Read the model definition and answer for the solid it produces. Units are mm, in the model's axes. Face numbers are marked on the shaded views. A direction names the side the tool comes from. Round coordinates to 2 decimals unless told otherwise and drop trailing zeros. Loops run counter-clockwise (first coordinate to the right, second up) from the corner with the lowest first, then second, coordinate; pieces in that order, holes last. Notation, with made-up numbers: M 58.5,32.25 L 115.5,32.25 A18 cw 115.5,36.25 Z; hole C 6.5,83 d4. An arc over 180 degrees is marked long. Write each question's results on one line, items separated by ' | '.
```python
from build123d import *

# Parameters (mm, degrees)
SKETCH1_R           = 205
SKETCH1_R_2         = 195
BOSS_EXTRUDE1_DEPTH = 110
CUT_EXTRUDE1_START  = 41.95
CUT_EXTRUDE1_DEPTH  = 26.1
BOSS_EXTRUDE3_DEPTH = 110
SKETCH5_R           = 10
CUT_EXTRUDE2_DEPTH  = 140
FILLET1_R           = 12.5
CUT_EXTRUDE4_START  = -7.5
CUT_EXTRUDE4_DEPTH  = 7.5
CUT_EXTRUDE5_DEPTH  = 7.5
FILLET2_R           = 12.5


with BuildPart() as part:
    # Sketch1 → Boss-Extrude1 (new body)
    with BuildSketch(Plane(origin=(0, 0, 0), x_dir=(0, 0, -1), z_dir=(1, 0, 0))):
        Circle(SKETCH1_R)
        Circle(SKETCH1_R_2, mode=Mode.SUBTRACT)
    extrude(amount=BOSS_EXTRUDE1_DEPTH)

    # Sketch3 → Cut-Extrude1 (cut)
    with BuildSketch(Plane(origin=(0, 0, 0), x_dir=(0, 0, -1), z_dir=(1, 0, 0)).offset(CUT_EXTRUDE1_START)):
        with BuildLine():
            Line((160.8479694, 127.09418059), (137.885822331, 137.885822331))
            ThreePointArc((137.885822331, 137.885822331), (143.004745144, 132.569388874), (147.918824855, 127.063060145))
            Line((147.918824855, 127.063060145), (167.43543162, 118.280920855))
            ThreePointArc((167.43543162, 118.280920855), (164.200841146, 122.731755332), (160.8479694, 127.09418059))
        make_face()
    extrude(amount=CUT_EXTRUDE1_DEPTH, mode=Mode.SUBTRACT)

    # Sketch4 → Boss-Extrude3 (add)
    with BuildSketch(Plane.ZY):
        with BuildLine():
            Line((-339.535373084, 38.097443801), (-170.172659449, 114.307768661))
            ThreePointArc((-170.172659449, 114.307768661), (-156.650879802, -132.232756371), (84.122100255, -186.945104907))
            Line((84.122100255, -186.945104907), (-183.982931916, -307.587784512))
            Line((-183.982931916, -307.587784512), (-339.535373084, 38.097443801))
        make_face()
    extrude(amount=-BOSS_EXTRUDE3_DEPTH)

    # Sketch5 → Cut-Extrude2 (cut)
    with BuildSketch(Plane(origin=(0, -120.642679605, -268.105032171), x_dir=(-1, 0, 0), z_dir=(0, -0.41035170855993064, -0.9119273410102067))):
        with Locations(Location((-90, -185, 0), (0, 0, 90))):
            Circle(SKETCH5_R)
        with Locations(Location((-20, -185, 0), (0, 0, 90))):
            Circle(SKETCH5_R)
        with Locations(Location((-20, 154.071021086, 0), (0, 0, 90))):
            Circle(SKETCH5_R)
        with Locations(Location((-90, 154.071021086, 0), (0, 0, 90))):
            Circle(SKETCH5_R)
    extrude(amount=-CUT_EXTRUDE2_DEPTH, mode=Mode.SUBTRACT)

    # Fillet1
    fillet1_edges = [part.edges().sort_by_distance(p)[0] for p in [
        (55, 114.307768661, -170.172659449),
    ]]
    fillet(fillet1_edges, radius=FILLET1_R)

    # Sketch6 → Cut-Extrude4 (cut)
    with BuildSketch(Plane(origin=(110, 0, 0), x_dir=(0, 0, -1), z_dir=(1, 0, 0)).offset(CUT_EXTRUDE4_START)):
        with BuildLine():
            Line((326.312582588, 33.081687477), (179.407480032, 99.186471399))
            ThreePointArc((179.407480032, 99.186471399), (170.629059775, -113.625366712), (-22.343234006, -203.778752313))
            Line((-22.343234006, -203.778752313), (178.967175591, -294.364994017))
            Line((178.967175591, -294.364994017), (326.312582588, 33.081687477))
        make_face()
    extrude(amount=CUT_EXTRUDE4_DEPTH, mode=Mode.SUBTRACT)

    # Sketch7 → Cut-Extrude5 (cut)
    with BuildSketch(Plane.ZY):
        with BuildLine():
            Line((-179.407480032, 99.186471399), (-326.312582588, 33.081687477))
            Line((-326.312582588, 33.081687477), (-178.967175591, -294.364994017))
            Line((-178.967175591, -294.364994017), (22.343234006, -203.778752313))
            ThreePointArc((22.343234006, -203.778752313), (-170.629059775, -113.625366712), (-179.407480032, 99.186471399))
        make_face()
    extrude(amount=-CUT_EXTRUDE5_DEPTH, mode=Mode.SUBTRACT)

    # Fillet2
    # the kernel refuses this fillet: 12.5 mm, written as the material it adds along each edge
    with BuildSketch(Plane(origin=(102.5, -192.025828775, 48.461834434), x_dir=(1, 0, 0), z_dir=(0, -0.4103517085599303, -0.9119273410102069))) as fillet2_piece_1_section:
        with BuildLine():
            CenterArc((12.5, -11.456439237), FILLET2_R, 113.578178478, 66.421821522)
            Line((0, -11.456439237), (0, 0))
            Line((0, 0), (7.5, 0))
        make_face()
    fillet2_piece_1 = extrude(amount=249.39378369, mode=Mode.PRIVATE)
    fillet2_piece_1 = fillet2_piece_1 - Plane(origin=(104.520833168, 0, 0), x_dir=(0, 0.4838364458471492, -0.8751584391811569), z_dir=(-1, 0, 0)) * Cylinder(205, 545, mode=Mode.PRIVATE)
    add(fillet2_piece_1)
    with BuildSketch(Plane(origin=(102.5, 0, 0), x_dir=(0, 0.6010821181754732, -0.7991872666713895), z_dir=(0, 0.7991872666713895, 0.6010821181754732))) as fillet2_piece_2_section:
        with BuildLine():
            CenterArc((216.456439237, -12.5), FILLET2_R, 90, 66.421821522)
            Line((216.456439237, 0), (205, 0))
            Line((205, 0), (205, -7.5))
        make_face()
    fillet2_piece_2 = revolve(axis=Axis((102.5, 0, 0), (-1, 0, 0)), revolution_arc=141.215785086, mode=Mode.PRIVATE)
    fillet2_piece_2 = split(fillet2_piece_2, bisect_by=Plane(origin=(104.520833168, -262.670858667, -108.533087047), z_dir=(0, 0.9119273410102068, -0.41035170855993025)), keep=Keep.TOP, mode=Mode.PRIVATE)
    fillet2_piece_2 = split(fillet2_piece_2, bisect_by=Plane(origin=(104.520833168, 64.775822826, -255.878494044), z_dir=(0, -0.9119273410102069, 0.41035170855993014)), keep=Keep.TOP, mode=Mode.PRIVATE)
    add(fillet2_piece_2)
    with BuildSketch(Plane(origin=(102.5, 33.081687477, -326.312582588), x_dir=(1, 0, 0), z_dir=(0, 0.41035170855993014, 0.9119273410102069))) as fillet2_piece_3_section:
        with BuildLine():
            CenterArc((12.5, -11.456439237), FILLET2_R, 113.578178478, 66.421821522)
            Line((0, -11.456439237), (0, 0))
            Line((0, 0), (7.5, 0))
        make_face()
    fillet2_piece_3 = extrude(amount=189.734088675, mode=Mode.PRIVATE)
    fillet2_piece_3 = fillet2_piece_3 - Plane(origin=(104.520833168, 0, 0), x_dir=(0, 0.4838364458471492, -0.8751584391811569), z_dir=(-1, 0, 0)) * Cylinder(205, 426, mode=Mode.PRIVATE)
    add(fillet2_piece_3)
    with BuildSketch(Plane(origin=(102.5, -294.364994017, -178.967175591), x_dir=(1, 0, 0), z_dir=(0, 0.9119273410102068, -0.4103517085599305)), Plane(origin=(7.5, 33.081687477, -326.312582588), x_dir=(-1, 0, 0), z_dir=(0, -0.9119273410102068, 0.41035170855993064))) as fillet2_piece_4:
        with BuildLine():
            CenterArc((12.5, -11.456439237), FILLET2_R, 113.578178478, 66.421821522)
            Line((0, -11.456439237), (0, 0))
            Line((0, 0), (7.5, 0))
        make_face()
    extrude(amount=359.071021086)
    with BuildSketch(Plane(origin=(7.5, -294.364994017, -178.967175591), x_dir=(-1, 0, 0), z_dir=(0, 0.41035170855993075, 0.9119273410102067))) as fillet2_piece_5_section:
        with BuildLine():
            CenterArc((12.5, -11.456439237), FILLET2_R, 113.578178478, 66.421821522)
            Line((0, -11.456439237), (0, 0))
            Line((0, 0), (7.5, 0))
        make_face()
    fillet2_piece_5 = extrude(amount=249.39378369, mode=Mode.PRIVATE)
    fillet2_piece_5 = fillet2_piece_5 - Plane(origin=(5.479166832, 0, 0), x_dir=(0, 0, -1), z_dir=(-1, 0, 0)) * Cylinder(195, 545, mode=Mode.PRIVATE)
    add(fillet2_piece_5)
    with BuildSketch(Plane(origin=(7.5, 110.939394936, -153.288879604), x_dir=(-1, 0, 0), z_dir=(0, -0.4103517085599306, -0.9119273410102067))) as fillet2_piece_6_section:
        with BuildLine():
            CenterArc((12.5, -11.456439237), FILLET2_R, 113.578178478, 66.421821522)
            Line((0, -11.456439237), (0, 0))
            Line((0, 0), (7.5, 0))
        make_face()
    fillet2_piece_6 = extrude(amount=189.734088675, mode=Mode.PRIVATE)
    fillet2_piece_6 = fillet2_piece_6 - Plane(origin=(5.479166832, 0, 0), x_dir=(0, 0, -1), z_dir=(-1, 0, 0)) * Cylinder(195, 426, mode=Mode.PRIVATE)
    add(fillet2_piece_6)
    with BuildSketch(Plane(origin=(7.5, 0, 0), x_dir=(0, -0.9691520376470129, 0.24646364422495046), z_dir=(0, 0.24646364422495046, 0.9691520376470129))) as fillet2_piece_7_section:
        with BuildLine():
            CenterArc((216.456439237, -12.5), FILLET2_R, 90, 66.421821522)
            Line((216.456439237, 0), (205, 0))
            Line((205, 0), (205, -7.5))
        make_face()
    fillet2_piece_7 = revolve(axis=Axis((7.5, 0, 0), (1, 0, 0)), revolution_arc=141.215785086, mode=Mode.PRIVATE)
    fillet2_piece_7 = split(fillet2_piece_7, bisect_by=Plane(origin=(5.479166832, -262.670858667, -108.533087047), z_dir=(0, 0.9119273410102067, -0.41035170855993075)), keep=Keep.TOP, mode=Mode.PRIVATE)
    fillet2_piece_7 = split(fillet2_piece_7, bisect_by=Plane(origin=(5.479166832, 64.775822826, -255.878494044), z_dir=(0, -0.9119273410102067, 0.4103517085599306)), keep=Keep.TOP, mode=Mode.PRIVATE)
    add(fillet2_piece_7)


solid = part.part
```
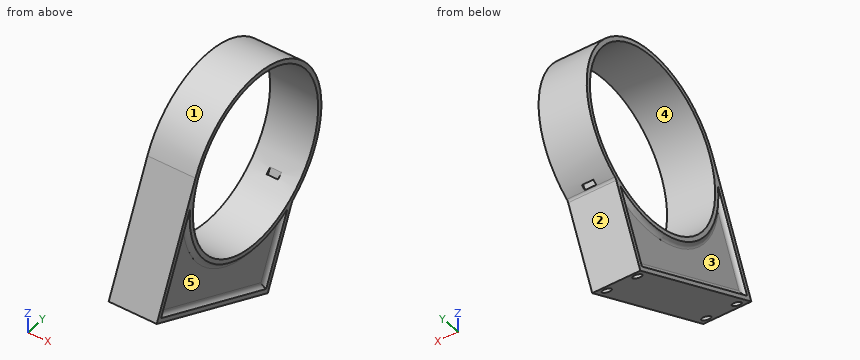
1. Which of the six approach directions +Z, -Z, +X, -X, +Y, -Y give full straight-line access (tool end or side, diameter ignored) to the marked faces 4 and 5?
Completed:
face 4: +X, -X | face 5: +X
2. Determine the mould class of the marked faces 1, 2 and 3 for opening direction Y: released by +Y, released by -Y, zero draft, split by the parting line, or undercut.
Completed:
face 1: split by the parting line | face 2: released by +Y | face 3: undercut
3. Find section B-B, the plane z = -130.5. Count the separate pieces of the cut face and the enclosed holes in it, then the cut area to 3 significant figures.
Completed:
separate pieces: 2 | enclosed holes: 2 | area: 14,400 mm2
4. Find the intervals of material crossed by L1, parallel to Y at x = 82.5, z = -91; L2, parallel to Z at x = 72, y = 0; L3, parallel to Z at x = 81.5, y = 5.5, in increasing order.
Completed:
L1: y = -265.75 to -251.07, -236.56 to -172.46, 172.46 to 183.7 | L2: z = -322.39 to -195, 195 to 205 | L3: z = -324.87 to -194.92, 194.92 to 204.93
5. Find section A-A, the plane x = 59. Give the vertices of the cut face in (y, z).
Completed:
outline: M -307.59,-183.98 L 38.1,-339.54 L 112.87,-173.38 A12.5 cw 117.12,-168.25 A205 ccw 118.28,-167.44 L 127.06,-147.92 A195 cw long 137.89,-137.89 L 127.09,-160.85 A205 ccw long -186.95,84.12 Z
6. Given P1, Ø4, axis at x = 50.5, y = 9, coming from the -Z side; P2, Ø3, axis at x = 20.5, y = -91.5, coming from the -Z side; P3, Ø3, axis at x = 77, y = 57.5, coming from the +Z side, each flat-ended and moving along its own axis, determine where each tip first touches the part or whether it passes through.
Completed:
P1: stops at z = -327.34 | P2: stops at z = -281.89 | P3: stops at z = 197.2
